For this review, take the finished solid that the model builds, in its own axes (mm). A direction names the side the tool comes from. Give positions to 0.01 mm unless a question says otherwise; leave off trailing zeros. Loops run counter-clockwise (first coordinate to the right, second up) from the corner with the lowest first, then second, coordinate; pieces in that order, holes last.
```python
from build123d import *

# Parameters (mm, degrees)
TUBE_EXTRUDE_DEPTH                                  = 25
UPPER_START                                         = 3
PIN_RING_SKETCH_R                                   = 12.5
PIN_RING_SKETCH_R_2                                 = 10
UPPER_RIGHT_PIN_RING_EXTRUDE_DEPTH                  = 3
LOWER_START                                         = -3
PIN_RING_SKETCH_2_R                                 = 12.5
PIN_RING_SKETCH_2_R_2                               = 10
LOWER_RIGHT_PIN_RING_EXTRUDE_DEPTH                  = 3
UPPER_RIGHT_RING_CONNECTION_EXTRUDE_REACH           = 57.453
UPPER_RIGHT_RING_CONNECTION_EXTRUDE_END_RADIUS      = 35
UPPER_RIGHT_RING_CONNECTION_SKETCH_W                = 25
UPPER_RIGHT_RING_CONNECTION_SKETCH_H                = 3
UPPER_RIGHT_RING_CONNECTION_EXTRUDE_DIRE_REACH      = 57.453
UPPER_RIGHT_RING_CONNECTION_EXTRUDE_DIRE_END_RADIUS = 12.5
LOWER_RIGHT_RING_CONNECTION_EXTRUDE_REACH           = 57.453
LOWER_RIGHT_RING_CONNECTION_EXTRUDE_END_RADIUS      = 35
LOWER_RIGHT_RING_CONNECTION_SKETCH_W                = 25
LOWER_RIGHT_RING_CONNECTION_SKETCH_H                = 3
LOWER_RIGHT_RING_CONNECTION_EXTRUDE_DIRE_REACH      = 57.453
LOWER_RIGHT_RING_CONNECTION_EXTRUDE_DIRE_END_RADIUS = 12.5
FAULTY_START                                        = -35
FAULTY_MIRROR_DEPTH                                 = 70
FAULTY_START_2                                      = -25
FAULTY_MIRROR_2_DEPTH                               = 25
MIRROR_HACK_CUT_REACH                               = 78.851
MIRROR_HACK_SKETCH_R                                = 10


with BuildPart() as part:
    # Tube Sketch → Tube Extrude (new body)
    with BuildSketch(Plane.XY):
        with BuildLine():
            Line((0, 35), (0, 30))
            ThreePointArc((0, 30), (-30, 0), (0, -30))
            Line((0, -30), (0, -35))
            ThreePointArc((0, -35), (-35, 0), (0, 35))
        make_face()
    extrude(amount=-TUBE_EXTRUDE_DEPTH)



with BuildPart() as body_2:
    # Pin Ring Sketch → Upper Right Pin Ring Extrude (new body)
    with BuildSketch(Plane(origin=(0, 0, 0), x_dir=(1, 0, 0), z_dir=(0, 1, 0)).offset(UPPER_START)):
        with Locations(Location((-47.5, 12.5, 0), (0, 0, 270))):
            Circle(PIN_RING_SKETCH_R)
        with Locations(Location((-47.5, 12.5, 0), (0, 0, 270))):
            Circle(PIN_RING_SKETCH_R_2, mode=Mode.SUBTRACT)
    extrude(amount=UPPER_RIGHT_PIN_RING_EXTRUDE_DEPTH)


with BuildPart() as body_3:
    # Pin Ring Sketch<2> → Lower Right Pin Ring Extrude (new body)
    with BuildSketch(Plane(origin=(0, 0, 0), x_dir=(1, 0, 0), z_dir=(0, 1, 0)).offset(LOWER_START)):
        with Locations(Location((-47.5, 12.5, 0), (0, 0, 270))):
            Circle(PIN_RING_SKETCH_2_R)
        with Locations(Location((-47.5, 12.5, 0), (0, 0, 270))):
            Circle(PIN_RING_SKETCH_2_R_2, mode=Mode.SUBTRACT)
    extrude(amount=-LOWER_RIGHT_PIN_RING_EXTRUDE_DEPTH)


with BuildPart() as part_1:
    add(part.part)

    add(body_2.part)  # Upper Right Ring Connection Extrude merges body 2
    # Upper Right Ring Connection Extrude: up to this cylinder (the profile starts outside it)
    upper_right_ring_connection_extrude_end = Plane(origin=(0, 0, -12.5), z_dir=(0, 0, 1)) * Cylinder(UPPER_RIGHT_RING_CONNECTION_EXTRUDE_END_RADIUS, 185.906, mode=Mode.PRIVATE)
    # Upper Right Ring Connection Sketch → Upper Right Ring Connection Extrude (add, up to the surface)
    with BuildSketch(Plane.ZY.offset(35), mode=Mode.PRIVATE) as upper_right_ring_connection_extrude_sk1:
        with Locations((-12.5, 4.5)):
            Rectangle(UPPER_RIGHT_RING_CONNECTION_SKETCH_W, UPPER_RIGHT_RING_CONNECTION_SKETCH_H)
    upper_right_ring_connection_extrude_tool1 = extrude(upper_right_ring_connection_extrude_sk1.sketch, amount=-UPPER_RIGHT_RING_CONNECTION_EXTRUDE_REACH, mode=Mode.PRIVATE) - upper_right_ring_connection_extrude_end
    add(upper_right_ring_connection_extrude_tool1.solids().sort_by_distance((-35, 4.5, -12.5))[0])

    # Upper Right Ring Connection Extrude dire: up to this cylinder (the profile starts outside it)
    upper_right_ring_connection_extrude_dire_end = Plane(origin=(-47.5, 4.5, -12.5), z_dir=(0, -1, 0)) * Cylinder(UPPER_RIGHT_RING_CONNECTION_EXTRUDE_DIRE_END_RADIUS, 140.906, mode=Mode.PRIVATE)
    # Upper Right Ring Connection Sketch → Upper Right Ring Connection Extrude dire (add, up to the surface)
    with BuildSketch(Plane.ZY.offset(35), mode=Mode.PRIVATE) as upper_right_ring_connection_extrude_dire_sk1:
        with Locations((-12.5, 4.5)):
            Rectangle(UPPER_RIGHT_RING_CONNECTION_SKETCH_W, UPPER_RIGHT_RING_CONNECTION_SKETCH_H)
    upper_right_ring_connection_extrude_dire_tool1 = extrude(upper_right_ring_connection_extrude_dire_sk1.sketch, amount=UPPER_RIGHT_RING_CONNECTION_EXTRUDE_DIRE_REACH, mode=Mode.PRIVATE) - upper_right_ring_connection_extrude_dire_end
    add(upper_right_ring_connection_extrude_dire_tool1.solids().sort_by_distance((-35, 4.5, -12.5))[0])
    add(upper_right_ring_connection_extrude_dire_tool1.solids().sort_by_distance((-35, 4.5, -12.5))[1])


    add(body_3.part)  # Lower Right Ring Connection Extrude merges body 3
    # Lower Right Ring Connection Extrude: up to this cylinder (the profile starts outside it)
    lower_right_ring_connection_extrude_end = Plane(origin=(0, 0, -12.5), z_dir=(0, 0, 1)) * Cylinder(LOWER_RIGHT_RING_CONNECTION_EXTRUDE_END_RADIUS, 185.906, mode=Mode.PRIVATE)
    # Lower Right Ring Connection Sketch → Lower Right Ring Connection Extrude (add, up to the surface)
    with BuildSketch(Plane.ZY.offset(35), mode=Mode.PRIVATE) as lower_right_ring_connection_extrude_sk1:
        with Locations((-12.5, -4.5)):
            Rectangle(LOWER_RIGHT_RING_CONNECTION_SKETCH_W, LOWER_RIGHT_RING_CONNECTION_SKETCH_H)
    lower_right_ring_connection_extrude_tool1 = extrude(lower_right_ring_connection_extrude_sk1.sketch, amount=-LOWER_RIGHT_RING_CONNECTION_EXTRUDE_REACH, mode=Mode.PRIVATE) - lower_right_ring_connection_extrude_end
    add(lower_right_ring_connection_extrude_tool1.solids().sort_by_distance((-35, -4.5, -12.5))[0])

    # Lower Right Ring Connection Extrude dire: up to this cylinder (the profile starts outside it)
    lower_right_ring_connection_extrude_dire_end = Plane(origin=(-47.5, -4.5, -12.5), z_dir=(0, 1, 0)) * Cylinder(LOWER_RIGHT_RING_CONNECTION_EXTRUDE_DIRE_END_RADIUS, 140.906, mode=Mode.PRIVATE)
    # Lower Right Ring Connection Sketch → Lower Right Ring Connection Extrude dire (add, up to the surface)
    with BuildSketch(Plane.ZY.offset(35), mode=Mode.PRIVATE) as lower_right_ring_connection_extrude_dire_sk1:
        with Locations((-12.5, -4.5)):
            Rectangle(LOWER_RIGHT_RING_CONNECTION_SKETCH_W, LOWER_RIGHT_RING_CONNECTION_SKETCH_H)
    lower_right_ring_connection_extrude_dire_tool1 = extrude(lower_right_ring_connection_extrude_dire_sk1.sketch, amount=LOWER_RIGHT_RING_CONNECTION_EXTRUDE_DIRE_REACH, mode=Mode.PRIVATE) - lower_right_ring_connection_extrude_dire_end
    add(lower_right_ring_connection_extrude_dire_tool1.solids().sort_by_distance((-35, -4.5, -12.5))[0])
    add(lower_right_ring_connection_extrude_dire_tool1.solids().sort_by_distance((-35, -4.5, -12.5))[1])

    # Faulty Mirror: read off the stored shape, not the designer's step
    # Faulty Mirror outline → Faulty Mirror (add)
    with BuildSketch(Plane(origin=(0, 0, 0), x_dir=(1, 0, 0), z_dir=(0, 1, 0)).offset(FAULTY_START)):
        with BuildLine():
            Line((47.5, 25), (0, 25))
            Line((0, 25), (0, 0))
            Line((0, 0), (47.5, 0))
            ThreePointArc((47.5, 0), (60, 12.5), (47.5, 25))
        make_face()
    extrude(amount=FAULTY_MIRROR_DEPTH)

    # Faulty Mirror 2 outline → Faulty Mirror 2 (cut)
    with BuildSketch(Plane.XY.offset(FAULTY_START_2)):
        with BuildLine():
            ThreePointArc((34.871191548, 3), (35, 0), (34.871191548, -3))
            Line((34.871191548, -3), (61, -3))
            Line((61, -3), (61, 3))
            Line((61, 3), (34.871191548, 3))
        make_face()
        with BuildLine():
            Line((61, -35), (61, -6))
            Line((61, -6), (34.481879299, -6))
            ThreePointArc((34.481879299, -6), (22.527760652, -26.786190472), (0, -35))
            Line((0, -35), (61, -35))
        make_face()
        with BuildLine():
            Line((34.481879299, 6), (61, 6))
            Line((61, 6), (61, 35))
            Line((61, 35), (0, 35))
            ThreePointArc((0, 35), (22.527760652, 26.786190472), (34.481879299, 6))
        make_face()
        with BuildLine():
            Line((0, 30), (0, -30))
            ThreePointArc((0, -30), (30, 0), (0, 30))
        make_face()
    extrude(amount=FAULTY_MIRROR_2_DEPTH, mode=Mode.SUBTRACT)

    # Mirror Hack Cut: up to this face of the body (flat: up to its plane)
    mirror_hack_cut_end = Plane(part_1.part.faces().sort_by_distance((46.070109689, -6, -12.5))[0])
    # Mirror Hack Sketch → Mirror Hack Cut (cut, up to the picked face)
    with BuildSketch(Plane(origin=(0, 6, 0), x_dir=(1, 0, 0), z_dir=(0, 1, 0)), mode=Mode.PRIVATE) as mirror_hack_cut_sk1:
        with Locations(Location((47.5, 12.5, 0), (0, 0, 270))):
            Circle(MIRROR_HACK_SKETCH_R)
    mirror_hack_cut_tool1 = split(extrude(mirror_hack_cut_sk1.sketch, amount=-MIRROR_HACK_CUT_REACH, mode=Mode.PRIVATE), bisect_by=mirror_hack_cut_end, keep=Keep.BOTH, mode=Mode.PRIVATE)
    add(mirror_hack_cut_tool1.solids().sort_by(Axis((47.5, 6, -12.5), (0, -1, 0)))[0], mode=Mode.SUBTRACT)


solid = part_1.part
```
Q1. Consider section B-B on y = -20.5. Give the boundary of the cut face in (x, z), plus the area to 3 significant figures.
Answers:
outline: (-28.37, -25) - (-21.9, -25) - (-21.9, 0) - (-28.37, 0) - close; (21.9, -25) - (28.37, -25) - (28.37, 0) - (21.9, 0) - close
area: 323 mm2
Q2. Machinability: for faces 5 (the flat face through (38.6, 6, -18.2)), 6 (the flat face through (-38.9, 3, -18.2)), 7 (the flat face through (38.9, -3, -18.2)), which of the approach directions +Z, -Z, +X, -X, +Y, -Y give a long, thin tool a straight path to every point of the face, cutting with its end or side? Answer none if there is none.
Answers:
face 5: +Z, -Z, +X, +Y
face 6: +Z, -Z, -X
face 7: +Z, -Z, +X
Q3. Consider section D-D on z = -12.5. Count the separate pieces of the cut face and the enclosed holes in it, plus the area to 3 significant figures.
Answers:
separate pieces: 5
enclosed holes: 1
area: 1,080 mm2
Q4. For pin 1 Ø1.5 at (y, z) = (-22, -12.5) entering from -X; pin 2 Ø2 at (x, z) = (-36, -6) entering from -Y; pin 3 Ø1 at (x, z) = (-16.5, -12.5) entering from -Y, all flat-tipped, find the tip position at first contact; note any pin that passes through.
Answers:
pin 1: stops at x = -27.81
pin 2: stops at y = -6
pin 3: stops at y = -31.13
Q5. Consider section A-A on x = -18. Give the boundary of the cut face in (y, z).
Answers:
outline: (-30.02, -25) - (-24, -25) - (-24, 0) - (-30.02, 0) - close; (24, -25) - (30.02, -25) - (30.02, 0) - (24, 0) - close
Q6. Mouldability with a two-part tool opening along Z and no side actions: class faces 1 (the flat face through (-38.9, -3, -18.2)), 2 (the cylindrical face through (37.74, -4.48, -14.67)), 3 (the cylindrical face through (59.997, -4.521, -12.225)), 4 (the flat face through (-28.4, -10.5, 0)) as +Z half, -Z half, draft (parallel to the pull), parting line (faces both ways), or undercut.
Answers:
face 1: draft
face 2: undercut
face 3: parting line
face 4: +Z half
Q7. Consider section C-C on x = -39. Give the boundary of the cut face in (y, z).
Answers:
outline: (-6, -25) - (-3, -25) - (-3, -17.77) - (-6, -17.77) - close; (-6, -7.23) - (-3, -7.23) - (-3, 0) - (-6, 0) - close; (3, -25) - (6, -25) - (6, -17.77) - (3, -17.77) - close; (3, -7.23) - (6, -7.23) - (6, 0) - (3, 0) - close
Q8. For probe 1 along Y at (x, z) = (45, -1); probe 2 along X at (y, z) = (-3.7, -12.5); probe 3 along X at (y, z) = (-4.55, -12.5), list the stretches that pass through material, from the lowest coordinate up.
Answers:
probe 1: y = -6 to -3, 3 to 6
probe 2: x = -60 to -57.5, -37.5 to -29.77, 29.77 to 37.5, 57.5 to 60
probe 3: x = -60 to -57.5, -37.5 to -29.65, 29.65 to 37.5, 57.5 to 60
